Geometry: final body of the model. Coordinates: model frame, mm. Give positions to 0.01 mm unless a question says otherwise; leave off trailing zeros. Write each loop counter-clockwise with the first axis right and the second up, starting at its lowest first coordinate (ties: lowest second). Pieces come first, ordered by that corner, then holes. Notation, with made-up numbers: (63.5, -10) -> (95.5, -10) arc R28 cw to (95.5, 29) -> close; hole circle Ø3 at (-24, 88.5). An arc over 180 degrees is marked (long way). Answer as a JSON object with one key per item and string values.
from build123d import *

# Parameters (mm, degrees)
F1_DEPTH = 95.25


with BuildPart() as f1:
    # F0 (on Front) → F1 (new body)
    with BuildSketch(Plane.XZ):
        with BuildLine():
            ThreePointArc((-13.855658, 2.178556), (-14.037455, 1.649547), (-14.09905, 1.093573))
            Line((-14.09905, 1.093573), (-14.09905, -9.595976))
            ThreePointArc((-14.09905, -9.595976), (-14.03879, -10.145966), (-13.86087, -10.669859))
            ThreePointArc((-13.86087, -10.669859), (-3.166244, -17.617713), (7.771441, -11.059152))
            ThreePointArc((7.771441, -11.059152), (7.979193, -10.497663), (8.04975, -9.903145))
            Line((8.04975, -9.903145), (8.04975, 1.320869))
            ThreePointArc((8.04975, 1.320869), (7.980533, 1.909795), (7.776653, 2.466623))
            ThreePointArc((7.776653, 2.466623), (-3.129417, 9.074671), (-13.855658, 2.178556))
        make_face()
    extrude(amount=F1_DEPTH)


solid = f1.part
Q1. First-contact query: P1, Ø1.5, axis at x = -11, y = -25.5, coming from the +Z side; P2, Ø2, axis at x = 1.5, y = -51, coming from the +Z side; P3, Ø2, axis at y = -47, z = -11, coming from the -X side. Flat tips, straight axial feed; report the tip coordinate or a pass-through.
Values:
{"P1": "z = 6.62", "P2": "z = 8.57", "P3": "x = -14.07"}
Q2. Cut plane B-B (z = 3.75). Return the cut outline in (x, y).
Values:
{"outline": "(-12.96, -95.25) -> (7.03, -95.25) -> (7.03, 0) -> (-12.96, 0) -> close"}
Q3. Material intervals for L1, parallel to Z at x = -4.5, y = -75.5; L2, parallel to Z at x = -4.75, y = -56.5; L3, parallel to X at y = -66, z = -11.75, sorted ascending. Write a range as from..to.
Values:
{"L1": "-17.52..8.98", "L2": "-17.48..8.94", "L3": "-13.29..7.39"}
Q4. Cut plane A-A (y = -77.5). Return the cut outline in (x, z).
Values:
{"outline": "(-14.1, -9.6) arc R2.54 ccw to (-13.86, -10.67) arc R12.04 ccw to (7.77, -11.06) arc R2.54 ccw to (8.05, -9.9) -> (8.05, 1.32) arc R2.54 ccw to (7.78, 2.47) arc R12.04 ccw to (-13.86, 2.18) arc R2.54 ccw to (-14.1, 1.09) -> close"}
Q5. Cut plane C-C (x = -10). Return the cut outline in (y, z).
Values:
{"outline": "(-95.25, -15.34) -> (0, -15.34) -> (0, 6.81) -> (-95.25, 6.81) -> close"}
